Input: part model. Units: mm. Frame: model coordinates. Face numbers are marked on the shaded views. A direction names the side the tool comes from. Round coordinates to 2 decimals unless told otherwise and drop trailing zeros. Order: outer loops, then holes, each group sorted by start corner. A loop starts at its lowest first (then second) coordinate and runs counter-clockwise, first axis right, second up. Notation, with made-up numbers: M 55,71 L 106,71 A20 ccw 106,96 Z; hole C -16.75,-25.75 d1. An arc over 180 degrees is marked long. One line per question, with ' | ' between items.
Autodesk Inventor part; units mm, degrees
ref_plane "YZ Plane" through (0, 0, 0) normal (1, 0, 0) x (0, 1, 0)
ref_plane "XZ Plane" through (0, 0, 0) normal (0, 1, 0) x (-1, 0, 0)
ref_plane "XY Plane" through (0, 0, 0) normal (0, 0, 1) x (1, 0, 0)
sketch "スケッチ1" plane through (0, 0, 0) normal (0, 0, 1) x (1, 0, 0)
  line L0 (-8.15, -4.25) -> (8.15, -4.25)
  line L1 (8.15, -4.25) -> (8.15, 4.25)
  line L2 (8.15, 4.25) -> (-8.15, 4.25)
  line L3 (-8.15, 4.25) -> (-8.15, -4.25)
  line L4 (-8.15, -4.25) -> (8.15, 4.25) construction
  line L5 (8.15, -4.25) -> (-8.15, 4.25) construction
  point P0 (0, 0)
  dimension "d0" = 16.3
  dimension "d1" = 8.5
extrude "押し出し1" add sketch "スケッチ1" along normal blind 14.5
ref_plane "作業平面2" through (0, 0, 10.5) normal (0, 0, -1) x (-1, 0, 0)
sketch "スケッチ3" plane through (0, 0, 10.5) normal (0, 0, -1) x (-1, 0, 0)
  circle A0 centre (10.15, 0) radius 0.9
  line L0 (8.15, 4.25) -> (8.15, -4.25)
  line L1 (8.15, -4.25) -> (8.15, 4.25)
  line L2 (8.15, 4.25) -> (10.15, 4.25)
  line L3 (8.15, -4.25) -> (10.15, -4.25)
  line L4 (8.15, 4.25) -> (8.15, -4.25)
  arc A1 (10.15, -4.25) -> (10.15, 4.25) centre (6.6589, 0) ccw
  point P0 (0, 0)
  point P1 (8.15, 0)
  dimension "d11" = 1.8
  dimension "d12" = 2
  dimension "d13" = 5.5
extrude "押し出し3" add sketch "スケッチ3" against normal blind 0.8
mirror "ミラー1" about plane through (0, 0, 0) normal (1, 0, 0) of "押し出し3"
sketch "スケッチ4" plane through (8.15, -4.25, 0) normal (1, 0, 0) x (0, 0, -1)
  circle A0 centre (-0.9, 4.25) radius 0.3
  circle A1 centre (-0.9, 4.85) radius 0.3
  circle A2 centre (-0.9, 3.65) radius 0.3
  line L0 (0, 0) -> (0, 8.5)
  point P0 (0, 4.25)
  point P1 (0, 4.25)
  dimension "d16" = 0.6
  dimension "d18" = 0.9
extrude "押し出し4" add sketch "スケッチ4" along normal blind 0.8
chamfer "面取り1" distance 4 distance2 1.5 1 edges at (-8.15, 0, 14.5) measured on face at (2.7167, -1.4167, 14.5)
sketch "スケッチ5" plane through (0, 0, 10.5) normal (0, 0, -1) x (-1, 0, 0)
  point P0 (0, 0)
sketch "スケッチ6" plane through (0, 0, 14.5) normal (0, 0, 1) x (1, 0, 0)
  arc A0 (0.2944, -2.25) -> (0.2944, 2.25) centre (3.9, 0) ccw
  line L0 (8.15, 4.25) -> (-4.15, 4.25)
  line L1 (8.15, -4.25) -> (8.15, 4.25)
  line L2 (-4.15, -4.25) -> (8.15, -4.25)
  arc A1 (-0.6, 2.25) -> (-0.6, -2.25) centre (-0.6, 0) ccw
  line L3 (-0.6, 2.25) -> (0.2944, 2.25)
  line L4 (-0.6, -2.25) -> (0.2944, -2.25)
  point P0 (0, 0)
  dimension "d24" = 4.5
  dimension "d25" = 4.5
extrude "押し出し5" add sketch "スケッチ6" along normal blind 3 contours L4 A1 L3 A0
sketch "スケッチ7" plane through (0, 0, 17.5) normal (0, 0, 1) x (1, 0, 0)
  arc A0 (8.15, 0) -> (3.9, 4.25) centre (3.9, 0) ccw
  circle A1 centre (3.9, 0) radius 1.9
  point P0 (0, 0)
  dimension "d28" = 3.8
extrude "押し出し6" add sketch "スケッチ7" along normal blind 3
sketch "スケッチ8" plane through (0, 0, 17.5) normal (0, 0, 1) x (1, 0, 0)
  line L0 (-1.4, 0) -> (-0.5, 0) construction
  line L1 (-1.4, -1.05) -> (-0.5, -1.05)
  line L2 (-0.5, 1.05) -> (-1.4, 1.05)
  arc A0 (-1.4, 1.05) -> (-1.4, -1.05) centre (-1.4, 0) ccw
  arc A1 (-0.5, -1.05) -> (-0.5, 1.05) centre (-0.5, 0) ccw
  arc A2 (-0.6, 2.25) -> (-0.6, -2.25) centre (-0.6, 0) ccw
  point P0 (0, 0)
  point P1 (-0.95, 0)
  dimension "d31" = 2.1
  dimension "d32" = 3
  dimension "d33" = 0.8
extrude "押し出し7" add sketch "スケッチ8" along normal blind 0.8
fillet "フィレット1" radius 0.1 4 edges at (8.15, 0, 17.5) (-2.85, 0, 17.5) (-0.1528, 2.25, 17.5) (-0.1528, -2.25, 17.5)
properties part number "Servo"
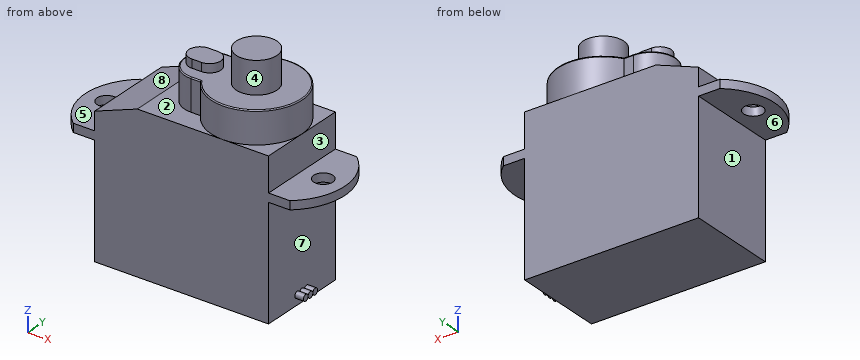
Item 1: Access query for the marked faces 1, 2, 3, 4 and 5. Directions: +Z, -Z, +X, -X, +Y, -Y. A direction counts if a zero-diameter tool reaches every point of the face in a straight line with its end or side. Return the directions, or none.
Report:
face 1: -Z, -X, +Y, -Y | face 2: +Z, -X | face 3: +Z, +X, +Y, -Y | face 4: +Z | face 5: +Z, -X, +Y, -Y
Item 2: First-contact query: pin 1 (0.7 mm diameter, centred on y = 0.5, z = 1, fed in from +X); pin 2 (1 mm diameter, centred on y = -1.5, z = 8, fed in from -X); pin 3 (1.6 mm diameter, centred on y = 0, z = 13.5, fed in from +X); pin 4 (4 mm diameter, centred on x = -5, z = 17.5, fed in from -Y). Flat tips, straight axial feed; report the tip coordinate or a pass-through.
Report:
pin 1: x = 8.95 | pin 2: x = -8.15 | pin 3: x = 8.15 | pin 4: through
Item 3: Mould query, pull axis Z, two halves, no side actions, for the marked faces 6, 7 and 8. Classes: +Z half, -Z half, draft (parallel to the pull), parting line (faces both ways), or undercut.
Report:
face 6: -Z half | face 7: undercut | face 8: +Z half
Item 4: Line query: line 1 along Y through (x, z) = (10.15, 10.75); line 2 along Z through (x, y) = (-4, -2.5); line 3 along X through (y, z) = (1.75, 9.75). Output: solid intervals per line, ascending. Write a range as from..to.
Report:
line 1: -4.25..-0.9, 0.9..4.25 | line 2: 0..14.5 | line 3: -8.15..8.15
Item 5: Section query A-A, the plane x = -7. Return loops of the section in (y, z), plus the area to 3 significant figures.
Report:
outline: M -4.25,0 L 4.25,0 L 4.25,13.43 L -4.25,13.43 Z | area: 114 mm²
